The listing builds one solid part. Answer for the finished solid, in the listing's coordinates (mm). A direction names the side the tool comes from. Give positions to 0.01 mm unless a question says otherwise; leave off trailing zeros. Write each loop counter-clockwise with the first axis right and the second up, starting at its lowest first coordinate (ties: lowest second). Pieces come first, ordered by that corner, then holes. Notation, with made-up numbers: (76.25, 4) - (135.25, 4) arc R17 ccw to (135.25, 28) - close; hole circle Ø6 at (-10, 77.5). An arc over 180 degrees is marked (long way). One line per question, with ' | ' between items. Start each with the question number.
1. Given P1, Ø6, axis at x = 6.5, y = 9.5, coming from the +Z side; P2, Ø0.8, axis at y = 4.5, z = -3.5, coming from the +X side; P3, Ø5, axis at x = -6.5, z = 1, coming from the +Y side, each flat-ended and moving along its own axis, determine where each tip first touches the part or whether it passes through.
2. For faces 1 (the face through (-0.1, 5.5, 4.5)), 2 (the face through (-3, 5, -4)), 3 (the face through (-5, 5, 3)), determine the directions among +Z, -Z, +X, -X, +Y, -Y from which every point of the face is accessible in a straight line to the end or side of a thin tool.
3. A cutting plane is placed at B-B (y = 9.5). Determine the outline of the cut face in (x, z), then the cut area to 3 significant figures.
4. Find the intervals of material crossed by L1, parallel to Y at x = 4, z = 1; L2, parallel to Y at x = -4.75, z = -3; L3, parallel to Z at x = -0.25, y = 19, in increasing order. Write a range as from..to.
5. A cutting plane is placed at A-A (y = 5). Determine the outline of the cut face in (x, z).
6. The mould has two halves that part along Y. Classify faces 4 (the face through (7.747, 1.232, -2.465)), 5 (the face through (7, 4, 0)), 6 (the face through (9.408, 3.26, 2.558)): +Y half, -Y half, draft (parallel to the pull), parting line (faces both ways), or undercut.
```python
from build123d import *

# Parameters (mm, degrees)
EXTRUDE_1_DEPTH     = 5
CUT_EXTRUDE_1_DEPTH = 1.5
SKETCH_2_R          = 4
EXTRUDE_2_DEPTH     = 25
CUT_EXTRUDE_2_DEPTH = 5
CHAMFER_2_SIZE      = 1


with BuildPart() as part:
    # Эскиз1 → Бобышка-Вытянуть1 (new body, symmetric)
    with BuildSketch(Plane.XY):
        Polygon((9.75, 0), (-9.75, 0), (-9.75, 4), (-5, 4), (-5, 5.5), (5, 5.5), (5, 4), (9.75, 4), align=None)
    extrude(amount=EXTRUDE_1_DEPTH, both=True)

    # Эскиз3 → Вырез-Вытянуть1 (cut)
    with BuildSketch(Plane(origin=(0, 5.5, 0), x_dir=(1, 0, 0), z_dir=(0, 1, 0))):
        with BuildLine():
            Line((-5, 0), (-5, 5))
            Line((-5, 5), (0, 5))
            ThreePointArc((0, 5), (-3.535533906, 3.535533906), (-5, 0))
        make_face()
        with BuildLine():
            Line((0, -5), (5, -5))
            Line((5, -5), (5, 0))
            ThreePointArc((5, 0), (3.535533906, -3.535533906), (0, -5))
        make_face()
    extrude(amount=-CUT_EXTRUDE_1_DEPTH, mode=Mode.SUBTRACT)

    # Эскиз2 → Бобышка-Вытянуть2 (add)
    with BuildSketch(Plane(origin=(0, 5.5, 0), x_dir=(1, 0, 0), z_dir=(0, 1, 0))):
        with Locations(Location((0, 0, 0), (0, 0, 270))):  # turned: the seam where the file's is
            Circle(SKETCH_2_R)
    extrude(amount=EXTRUDE_2_DEPTH)

    # Эскиз4 → Вырез-Вытянуть2 (cut, through all)
    with BuildSketch(Plane(origin=(0, 4, 0), x_dir=(1, 0, 0), z_dir=(0, 1, 0))):
        with BuildLine():
            Line((-8.370334521, 5), (-9.75, 5))
            Line((-9.75, 5), (-9.75, 0))
            ThreePointArc((-9.75, 0), (-9.398756875, 2.59342808), (-8.370334521, 5))
        make_face()
        with BuildLine():
            Line((8.370334521, -5), (9.75, -5))
            Line((9.75, -5), (9.75, 0))
            ThreePointArc((9.75, 0), (9.398756875, -2.59342808), (8.370334521, -5))
        make_face()
    extrude(amount=-CUT_EXTRUDE_2_DEPTH, mode=Mode.SUBTRACT)

    # Вырез-По траектории1: sweep along a path in Эскиз6
    with BuildLine(Plane.XZ) as sweep_1_path:
        Line((0, -9.75), (9.75, -9.75))
        Line((9.75, -9.75), (9.75, 0))
        ThreePointArc((9.75, 0), (6.894291117, 6.894291117), (0, 9.75))
        Line((0, 9.75), (-9.75, 9.75))
        Line((-9.75, 9.75), (-9.75, 0))
        ThreePointArc((-9.75, 0), (-6.894291117, -6.894291117), (0, -9.75))
    # Эскиз5 → Вырез-По траектории1 (sweep, cut)
    with BuildSketch(Plane.XY.offset(5)):
        Polygon((-9.75, 2.5), (-5.8, 0), (-9.75, 0), align=None)
    sweep(path=sweep_1_path.line, transition=Transition.RIGHT, mode=Mode.SUBTRACT)

    # Фаска2
    chamfer_2_edges = [part.edges().sort_by_distance(p)[0] for p in [
        (0, 30.5, -4),
    ]]
    chamfer(chamfer_2_edges, length=CHAMFER_2_SIZE)


solid = part.part
```
Determined:
1) P1: z = 1.94 | P2: x = 5 | P3: y = 5.5
2) face 1: +Y | face 2: -Z, -X, +Y | face 3: +Z, -Z, -X, +Y
3) outline: circle Ø8 at (0, 0) | area: 50.3 mm2
4) L1: 0..5.5 | L2: 0..4 | L3: -3.99..3.99
5) outline: (-5, 0) arc R5 ccw to (0, -5) - (5, -5) - (5, 0) arc R5 ccw to (0, 5) - (-5, 5) - close
6) face 4: -Y half | face 5: +Y half | face 6: draft
